Build history of the part. All positions in model axes, mm. A direction names the side the tool comes from. Give positions to 0.01 mm unless a question says otherwise; leave off trailing zeros. Answer in a Markdown table with one row per item.
```python
from build123d import *

# Parameters (mm, degrees)
F2_DEPTH = 700
F1_W     = 600
F1_H     = 550
F3_DEPTH = 800
F4_R     = 20
F5_R     = 245.6930164014
F6_DEPTH = 25
F7_R     = 24.99999


# Not quite as in the source:
# - a fillet or chamfer is up to 0.001 mm smaller than in the source, because OpenCascade refuses the exact size


with BuildPart() as f2:
    # F0 (on Top) → F2 (new body)
    with BuildSketch(Plane.XY):
        Polygon((81.1656415462, 504.1027583182), (-518.8343584538, 504.1027583182), (-518.8343584538, -45.8972416818), (-500.8343584538, -45.8972416818), (-500.8343584538, 501.1027583182), (63.1656415462, 501.1027583182), (63.1656415462, -45.8972416818), (81.1656415462, -45.8972416818), align=None)
    extrude(amount=F2_DEPTH)

    # F1 (on Top) → F3 (join)
    with BuildSketch(Plane.XY):
        with Locations((-218.8343584538, 229.1027583182)):
            Rectangle(F1_W, F1_H)
    extrude(amount=F3_DEPTH)

    # F4
    f4_edges = [f2.edges().sort_by_distance(p)[0] for p in [
        (-218.834358, -45.897242, 800),
        (81.165642, 229.102758, 800),
        (-518.834358, 229.102758, 800),
        (81.165642, -45.897242, 400),
        (-518.834358, -45.897242, 400),
    ]]
    fillet(f4_edges, radius=F4_R)

    # F5 (on face) → F6 (join)
    with BuildSketch(Plane.XZ.offset(45.8972416818)):
        with Locations((-218.8343584538, 390)):
            Circle(F5_R)
    extrude(amount=F6_DEPTH)

    # F7 (radius 25 in the source; OpenCascade refuses exactly that, so slightly less here)
    f7_edges = [f2.edges().sort_by_distance(p)[0] for p in [
        (-464.527375, -70.897242, 390),
    ]]
    fillet(f7_edges, radius=F7_R)


solid = f2.part
```
1. Drop flat-ended pins along their axis: P1, Ø3, axis at x = -112.5, z = 614, coming from the -Y side; P2, Ø10, axis at x = -250.5, z = 160.5, coming from the -Y side. Give the stop position or say it passes through.
Check result:
| item | result |
|---|---|
| P1 | stops at y = -45.9 |
| P2 | stops at y = -70.17 |
2. Probe line 1 (Y direction, x = -391.5, z = 157.5); line 2 (X direction, y = -39, z = 512.5). List the from-to ranges inside material, lowest first.
Check result:
| item | result |
|---|---|
| line 1 | y = -45.9 to 504.1 |
| line 2 | x = -513.94 to 76.28 |
3. Which spindle directions (+Z, -Z, +X, -X, +Y, -Y) get a long thin tool onto all of the face, cutting with end or side? Do faces 1 (the face through (-223, 233, 0)), 2 (the face through (-472, -45.897, 385)). Say none if no direction does.
Check result:
| item | result |
|---|---|
| face 1 | -Z, +X, -X, +Y, -Y |
| face 2 | -Y |
